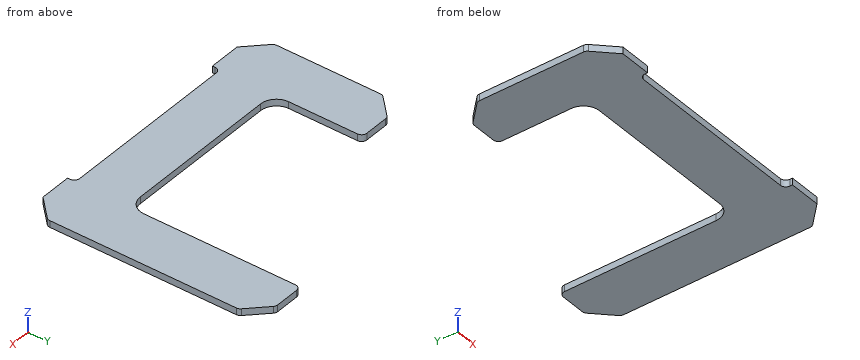
```python
from build123d import *

# Parameters (mm, degrees)
BOSS_EXTRUDE1_DEPTH      = 3.175
BOSS_EXTRUDE1_DEPTH_BACK = 3.175
CHAMFER1_SIZE            = 20
FILLET1_R                = 15
FILLET2_R                = 5


with BuildPart() as part:
    # Sketch2 → Boss-Extrude1 (new body, two sides)
    with BuildSketch(Plane.XY) as boss_extrude1_sk:
        Polygon((-138.5, 85.338455572), (-88.5, 85.338455572), (-88.5, 0), (88.5, 0), (88.5, 164), (138.5, 164), (138.5, -57.5), (88.5, -57.5), (88.5, -50), (-88.5, -50), (-88.5, -57.5), (-138.5, -57.5), align=None)
    extrude(amount=BOSS_EXTRUDE1_DEPTH)
    extrude(boss_extrude1_sk.sketch, amount=-BOSS_EXTRUDE1_DEPTH_BACK)

    # Chamfer1
    chamfer1_edges = [part.edges().sort_by_distance(p)[0] for p in [
        (-138.5, 85.338455572, 0),
        (138.5, 164, 0),
        (138.5, -57.5, 0),
        (-138.5, -57.5, 0),
    ]]
    chamfer(chamfer1_edges, length=CHAMFER1_SIZE)

    # Fillet1
    fillet1_edges = [part.edges().sort_by_distance(p)[0] for p in [
        (-88.5, 0, 0),
        (88.5, 0, 0),
    ]]
    fillet(fillet1_edges, radius=FILLET1_R)

    # Fillet2
    fillet2_edges = [part.edges().sort_by_distance(p)[0] for p in [
        (-88.5, 85.338455572, 0),
        (88.5, 164, 0),
        (88.5, -50, 0),
        (-88.5, -50, 0),
        (-138.5, 65.338455572, 0),
        (-138.5, -37.5, 0),
        (138.5, 144, 0),
        (138.5, -37.5, 0),
        (118.5, 164, 0),
        (-118.5, 85.338455572, 0),
    ]]
    fillet(fillet2_edges, radius=FILLET2_R)


solid = part.part
```
Verification items for the finished model (mm, model axes). Round coordinates to 2 decimals unless told otherwise and drop trailing zeros. Write each loop counter-clockwise with the first axis right and the second up, starting at its lowest first coordinate (ties: lowest second). Pieces come first, ordered by that corner, then holes.
1. Section check C-C on x = -107. Enter the section's corners in (y, z) (3 decimals).
2. Scan lines: L1, parallel to X at y = 24, z = -1; L2, parallel to Y at x = -3.5, z = 2.75; L3, parallel to X at y = 131, z = -2.25. Record each from-to range of solid material in increasing order.
3. Section check D-D on y = 105.5. Enter the section's corners in (x, z) (3 decimals), plus the area to 4 significant figures.
4. Section check B-B on z = -1. Enter the section's corners in (x, y).
5. Gauge pin test, flat ends, axial feed: P1, Ø1.9, axis at x = 1.5, z = 1, coming from the +Y side; P2, Ø3, axis at y = -55.5, z = -0.5, coming from the -X side; P3, Ø1.5, axis at x = 55, z = -1.5, coming from the -Y side. Record the tip position at first contact, or that the pin passes through.
6. Section check A-A on y = 48. Enter the section's corners in (x, z) (3 decimals), plus the area to 3 significant figures.
Answer:
1. outline: (-57.5, -3.175) - (85.338, -3.175) - (85.338, 3.175) - (-57.5, 3.175) - close
2. L1: x = -138.5 to -88.5, 88.5 to 138.5
2. L2: y = -50 to 0
2. L3: x = 88.5 to 138.5
3. outline: (88.5, -3.175) - (138.5, -3.175) - (138.5, 3.175) - (88.5, 3.175) - close
3. area: 317.5 mm2
4. outline: (-138.5, -35.43) arc R5 ccw to (-137.04, -38.96) - (-118.5, -57.5) - (-88.5, -57.5) - (-88.5, -55) arc R5 cw to (-83.5, -50) - (83.5, -50) arc R5 cw to (88.5, -55) - (88.5, -57.5) - (118.5, -57.5) - (137.04, -38.96) arc R5 ccw to (138.5, -35.43) - (138.5, 141.93) arc R5 ccw to (137.04, 145.46) - (119.96, 162.54) arc R5 ccw to (116.43, 164) - (93.5, 164) arc R5 ccw to (88.5, 159) - (88.5, 15) arc R15 cw to (73.5, 0) - (-73.5, 0) arc R15 cw to (-88.5, 15) - (-88.5, 80.34) arc R5 ccw to (-93.5, 85.34) - (-116.43, 85.34) arc R5 ccw to (-119.96, 83.87) - (-137.04, 66.8) arc R5 ccw to (-138.5, 63.27) - close
5. P1: stops at y = 0
5. P2: stops at x = -122
5. P3: stops at y = -50
6. outline: (-138.5, -3.175) - (-88.5, -3.175) - (-88.5, 3.175) - (-138.5, 3.175) - close; (88.5, -3.175) - (138.5, -3.175) - (138.5, 3.175) - (88.5, 3.175) - close
6. area: 635 mm2
